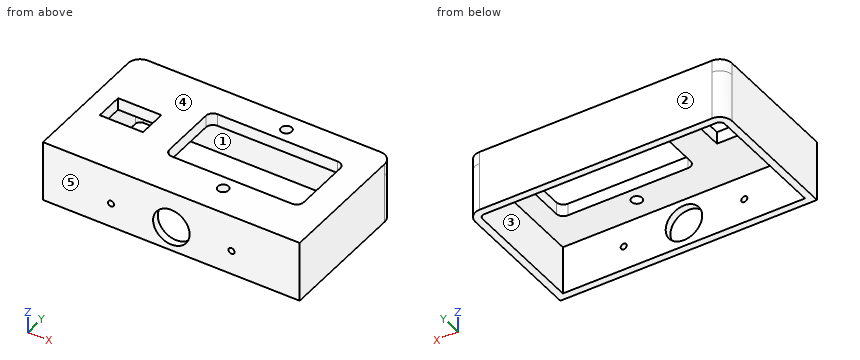
from build123d import *

# Parameters (mm, degrees)
ESBO_O1_W                                      = 105.544372836
ESBO_O1_H                                      = 58.736189027
ESBO_O1_R                                      = 2.2
RESSALTO_EXTRUS_O1_DEPTH                       = 5
ESBO_O2_W                                      = 17.8
ESBO_O2_H                                      = 11.6
CORTE_EXTRUS_O1_DEPTH                          = 10
FILETE1_R                                      = 5
RESSALTO_EXTRUS_O2_DEPTH                       = 20
BROCA_DE_ROSQUEAR_PARA_TARRAXA_DE_M3X0_5_D     = 2.5
BROCA_DE_ROSQUEAR_PARA_TARRAXA_DE_M3X0_5_DEPTH = 3
ESBO_O4_R                                      = 7.5
CORTE_EXTRUS_O2_DEPTH                          = 10


with BuildPart() as part:
    # Esboço1 → Ressalto-extrusão1 (new body)
    with BuildSketch(Plane.XY):
        with Locations((4.903986461, -60.193985815)):
            Rectangle(ESBO_O1_W, ESBO_O1_H)
        with Locations((18.576172879, -37.825891301)):
            Circle(ESBO_O1_R, mode=Mode.SUBTRACT)
        with Locations((18.576172879, -77.825891301)):
            Circle(ESBO_O1_R, mode=Mode.SUBTRACT)
        with BuildLine():
            Line((43.276172879, -43.425891301), (-6.123827121, -43.425891301))
            ThreePointArc((-6.123827121, -43.425891301), (-8.174436786, -44.275281636), (-9.023827121, -46.325891301))
            Line((-9.023827121, -46.325891301), (-9.023827121, -69.325891301))
            ThreePointArc((-9.023827121, -69.325891301), (-8.174436786, -71.376500966), (-6.123827121, -72.225891301))
            Line((-6.123827121, -72.225891301), (43.276172879, -72.225891301))
            ThreePointArc((43.276172879, -72.225891301), (45.326782544, -71.376500966), (46.176172879, -69.325891301))
            Line((46.176172879, -69.325891301), (46.176172879, -46.325891301))
            ThreePointArc((46.176172879, -46.325891301), (45.326782544, -44.275281636), (43.276172879, -43.425891301))
        make_face(mode=Mode.SUBTRACT)
    extrude(amount=RESSALTO_EXTRUS_O1_DEPTH)

    # Esboço2 → Corte-extrusão1 (cut)
    with BuildSketch(Plane.XY.offset(5)):
        with Locations((-30.968199957, -60.193985814)):
            Rectangle(ESBO_O2_W, ESBO_O2_H)
    extrude(amount=-CORTE_EXTRUS_O1_DEPTH, mode=Mode.SUBTRACT)

    # Filete1
    filete1_edges = [part.edges().sort_by_distance(p)[0] for p in [
        (-47.868199957, -30.825891301, 2.5),
        (57.676172879, -30.825891301, 2.5),
    ]]
    fillet(filete1_edges, radius=FILETE1_R)

    # Esboço3 → Ressalto-extrusão2 (add)
    with BuildSketch(Plane(origin=(0, 0, 0), x_dir=(-1, 0, 0), z_dir=(0, 0, -1))):
        with BuildLine():
            Line((42.868199957, -30.825891301), (-52.676172879, -30.825891301))
            ThreePointArc((-52.676172879, -30.825891301), (-56.211706785, -32.290357395), (-57.676172879, -35.825891301))
            Line((-57.676172879, -35.825891301), (-57.676172879, -89.562080328))
            Line((-57.676172879, -89.562080328), (47.868199957, -89.562080328))
            Line((47.868199957, -89.562080328), (47.868199957, -35.825891301))
            ThreePointArc((47.868199957, -35.825891301), (46.403733863, -32.290357395), (42.868199957, -30.825891301))
        make_face()
        with BuildLine():
            Line((42.868199957, -33.825891301), (-52.676172879, -33.825891301))
            ThreePointArc((-52.676172879, -33.825891301), (-54.090386441, -34.411677739), (-54.676172879, -35.825891301))
            Line((-54.676172879, -35.825891301), (-54.676172879, -86.562080328))
            Line((-54.676172879, -86.562080328), (44.868199957, -86.562080328))
            Line((44.868199957, -86.562080328), (44.868199957, -35.825891301))
            ThreePointArc((44.868199957, -35.825891301), (44.282413519, -34.411677739), (42.868199957, -33.825891301))
        make_face(mode=Mode.SUBTRACT)
    extrude(amount=RESSALTO_EXTRUS_O2_DEPTH)

    # Broca de rosquear para tarraxa de M3x0.51
    with Locations(Plane(origin=(0, -86.562080328, 0), x_dir=(1, 0, 0), z_dir=(0, 1, 0))):
        with Locations((29.645811084, 10.02860531), (-19.913744381, 10.02860531)):
            Hole(BROCA_DE_ROSQUEAR_PARA_TARRAXA_DE_M3X0_5_D / 2, depth=BROCA_DE_ROSQUEAR_PARA_TARRAXA_DE_M3X0_5_DEPTH)

    # Esboço4 → Corte-extrusão2 (cut)
    with BuildSketch(Plane(origin=(0, -86.562080328, 0), x_dir=(1, 0, 0), z_dir=(0, 1, 0))):
        with Locations((4.903986461, 10)):
            Circle(ESBO_O4_R)
    extrude(amount=-CORTE_EXTRUS_O2_DEPTH, mode=Mode.SUBTRACT)


solid = part.part
The listing builds one solid part. Answer for the finished solid, in the listing's coordinates (mm). Face numbers are marked on the shaded views. A direction names the side the tool comes from. Give positions to 0.01 mm unless a question says otherwise; leave off trailing zeros. Order: outer loops, then holes, each group sorted by start corner. A loop starts at its lowest first (then second) coordinate and runs counter-clockwise, first axis right, second up. Notation, with made-up numbers: (77, 59) - (119, 59) arc R19 ccw to (119, 77) - close; hole circle Ø10 at (-2.75, 68.5). An arc over 180 degrees is marked (long way). One line per item, written item: value. Start each with the question number.
1) A tool of negligible diameter and unlimited length cuts with its end or side. For the marked faces 1 and 2, from which of +Z, -Z, +X, -X, +Y, -Y can it reach the whole face along a straight path? Write none if from no direction.
2) A cutting plane is placed at D-D on z = -4.75. Give the vertices of the cut face in (x, y).
3) Find the intervals of material crossed by L1, parallel to X at y = -88.6, z = -10; L2, parallel to X at y = -58, z = 1.25; L3, parallel to X at y = -72.5, z = -0.5, in increasing order.
4) A cutting plane is placed at C-C on y = -49.5. Give the vertices of the cut face in (x, z).
5) A cutting plane is placed at A-A on y = -56. Give the vertices of the cut face in (x, z), then the cut area to 3 significant figures.
6) The mould has two halves that part along Y. Classify the marked faces 3, 4 and 5: released by +Y, released by -Y, zero draft, split by the parting line, or undercut.
7) Given pin 1 Ø2 at (x, z) = (29.65, -10.03) entering from -Y; pin 2 Ø5 at (x, y) = (18.58, -37.83) entering from +Z; pin 3 Ø6 at (x, y) = (-26.5, -75) entering from -Z, each flat-ended and moving along its own axis, determine where each tip first touches the part or whether it passes through.
8) A cutting plane is placed at B-B on x = 37.5. Give the vertices of the cut face in (y, z), then the cut area to 3 significant figures.
Answer sheet:
1. face 1: -Z
1. face 2: +Z, -Z, +X, -X, +Y
2. outline: (-47.87, -89.56) - (-0.45, -89.56) - (-0.45, -86.56) - (-44.87, -86.56) - (-44.87, -35.83) arc R2 cw to (-42.87, -33.83) - (52.68, -33.83) arc R2 cw to (54.68, -35.83) - (54.68, -86.56) - (10.26, -86.56) - (10.26, -89.56) - (57.68, -89.56) - (57.68, -35.83) arc R5 ccw to (52.68, -30.83) - (-42.87, -30.83) arc R5 ccw to (-47.87, -35.83) - close
3. L1: x = -47.87 to -21.16, -18.66 to -2.6, 12.4 to 28.4, 30.9 to 57.68
3. L2: x = -47.87 to -39.87, -22.07 to -9.02, 46.18 to 57.68
3. L3: x = -47.87 to -44.87, 54.68 to 57.68
4. outline: (-47.87, -20) - (-44.87, -20) - (-44.87, 0) - (-9.02, 0) - (-9.02, 5) - (-47.87, 5) - close; (46.18, 0) - (54.68, 0) - (54.68, -20) - (57.68, -20) - (57.68, 5) - (46.18, 5) - close
5. outline: (-47.87, -20) - (-44.87, -20) - (-44.87, 0) - (-39.87, 0) - (-39.87, 5) - (-47.87, 5) - close; (-22.07, 0) - (-9.02, 0) - (-9.02, 5) - (-22.07, 5) - close; (46.18, 0) - (54.68, 0) - (54.68, -20) - (57.68, -20) - (57.68, 5) - (46.18, 5) - close
5. area: 283 mm2
6. face 3: undercut
6. face 4: zero draft
6. face 5: released by -Y
7. pin 1: stops at y = -33.83
7. pin 2: stops at z = 5
7. pin 3: stops at z = 0
8. outline: (-89.56, -20) - (-86.56, -20) - (-86.56, 0) - (-72.23, 0) - (-72.23, 5) - (-89.56, 5) - close; (-43.43, 0) - (-33.83, 0) - (-33.83, -20) - (-30.83, -20) - (-30.83, 5) - (-43.43, 5) - close
8. area: 270 mm2
